Autodesk Fusion 360 part; units mm, degrees
sketch "Sketch1" plane through (0, 0, 0) normal (0, 0, 1) x (1, 0, 0)
  line L0 (50, 55) -> (66, 55) construction
  line L1 (50, 55) -> (34, 55) construction
  line L2 (50, 55) -> (50, 39) construction
  line L3 (50, 55) -> (50, 71) construction
  circle A0 centre (40.5, 55) radius 1.6
  circle A1 centre (50, 63) radius 1.6
  circle A2 centre (59.5, 55) radius 1.6
  circle A3 centre (50, 47) radius 1.6
  line L4 (65, 55) -> (66, 55)
  line L5 (35, 55) -> (34, 55)
  line L6 (50, 55) -> (46.1698, 51.7861) construction
  arc A4 (61.4907, 45.3582) -> (65, 55) centre (50, 55) ccw
  arc A5 (35, 55) -> (38.5093, 45.3582) centre (50, 55) ccw
  circle A6 centre (50, 55) radius 5
  line L7 (34, 55) -> (33.5, 55)
  line L8 (66, 55) -> (66.5, 55)
  circle A7 centre (50, 55) radius 15
  line L9 (50, 55) -> (53.8302, 51.7861) construction
  line L10 (61.4907, 45.3582) -> (62.2567, 44.7154) construction
  arc A8 (33.5, 55) -> (66.5, 55) centre (50, 55) ccw
  point P0 (59.5, 55)
  point P1 (50, 63)
  point P2 (50, 47)
  point P3 (40.5, 55)
  dimension "d23" = 30
  dimension "d25" = 8
  dimension "d26" = 8
  dimension "d27" = 9.5
  dimension "d28" = 9.5
  dimension "d29" = 3.2
  dimension "d30" = 3.2
  dimension "d31" = 3.2
  dimension "d32" = 3.2
  dimension "d33" = 140
  dimension "d34" = 80
  dimension "d41" = 10
  dimension "d44" = 33
extrude "Extrude7" add sketch "Sketch1" along normal blind 3 contours A4 A5 A7
extrude "Extrude8" add sketch "Sketch1" along normal blind 27 contours L4 L5 A4 A5 L7 L8 A7 A8
chamfer "Chamfer2" distance 0.5 distance2 2 1 edges at (45.3384, 56.8081, 3) measured on face at (42.065, 60.0544, 3)
chamfer "Chamfer3" distance 2 distance2 1 4 edges at (58.0083, 55.5786, 0) (48.5083, 47.5786, 0) (39.0083, 55.5786, 0) (48.5083, 63.5786, 0) measured on face at (60.434, 56.2991, 2) measured on face at (50.934, 48.2991, 2) measured on face at (41.434, 56.2991, 2) measured on face at (51.0587, 64.1997, 2)
fillet "Fillet1" radius 1.5 2 edges at (65, 55, 1.5) (35, 55, 1.5)
sketch "Sketch2" plane through (0, 0, 0) normal (0, 1, 0) x (1, 0, 0)
The model under review builds one solid part; all positions refer to its coordinate system, in mm. A direction names the side the tool comes from. Coordinates: 2 decimals unless noted, no trailing zeros. Write each loop counter-clockwise with the first axis right and the second up, starting at its lowest first coordinate (ties: lowest second). Pieces come first, ordered by that corner, then holes. Notation, with made-up numbers: (-18, 42.5) - (-14, 42.5) arc R23 cw to (-14, 51.5) - close; hole circle Ø10 at (86.25, -0.5). An arc over 180 degrees is marked (long way). Answer in a Markdown table with one row per item. Add a question column.
Q1. Consider section C-C on z = 19.75. Give the boundary of the cut face in (x, y).
Q2. To check wall thickness, follow line 1 along Y through (x, z) = (50, 2.6); line 2 along Y through (x, z) = (50, 0.35) (3 decimals); line 3 along Z through (x, y) = (58, 43.5). State the ranges of each line that lie inside material, in increasing order. Write a range as from..to.
Q3. Consider section A-A on x = 40.5. Give the boundary of the cut face in (y, z).
Q4. Clearance check with flat-ended pins moving along their axes: pin 1 (1.5 mm diameter, centred on y = 54.5, z = 18.5, fed in from +X); pin 2 (1.9 mm diameter, centred on x = 50, y = 47, fed in from +Z); pin 3 (6 mm diameter, centred on x = 55, z = 12.5, fed in from -Y); pin 4 (3.5 mm diameter, centred on x = 59.5, y = 55, fed in from +Z). State where each tip first meets the part, or that it passes through.
Q5. Draft analysis for pull direction Y (two halves, no side actions). For faces 1 (the face through (34.568, 55.382, 1.521)), 2 (the face through (53.4, 51, 0)), 3 (the face through (61.026, 54.519, 2.493)), 4 (the face through (49.349, 50.043, 0.493)), state which applies: +Y half, -Y half, draft (parallel to the pull), parting line (faces both ways), or undercut.
Q6. For faces 5 (the face through (57, 55, 3)), 6 (the face through (65.41, 55.4, 1.52)), list the 3-axis set-ups (+Z, -Z, +X, -X, +Y, -Y) from which the entire face can be reached by the end or side of a thin tool; tool diameter is ignored.
Q7. Consider section D-D on y = 47. Give the boundary of the cut face in (x, z).
Q8. Consider section B-B on y = 63. Give the boundary of the cut face in (x, z), then the cut area to 3 significant figures.
Answers below:
| question | item | result |
|---|---|---|
| 1 | outline | (33.5, 55) arc R16.5 ccw to (66.5, 55) - (65, 55) arc R15 cw to (61.49, 45.36) arc R15 cw to (38.51, 45.36) arc R15 cw to (35, 55) - close |
| 2 | line 1 | 38.5..45.4, 48.6..49.6, 60.4..61.4, 64.6..70 |
| 2 | line 2 | 38.5..44.575, 49.425..50, 60..60.575, 65.425..70 |
| 2 | line 3 | 0..3 |
| 3 | outline | (41.51, 0) - (52.4, 0) - (53.4, 2) - (53.4, 3) - (43.39, 3) - (43.39, 27) - (41.51, 27) - close; (56.6, 2) - (57.6, 0) - (66.61, 0) - (66.61, 3) - (56.6, 3) - close |
| 4 | pin 1 | x = 66.5 |
| 4 | pin 2 | through |
| 4 | pin 3 | y = 38.62 |
| 4 | pin 4 | z = 3 |
| 5 | face 1 | +Y half |
| 5 | face 2 | draft |
| 5 | face 3 | undercut |
| 5 | face 4 | undercut |
| 6 | face 5 | +Z, +Y |
| 6 | face 6 | +Z, -Z, +X, +Y |
| 7 | outline | (35.57, 0) - (47.4, 0) - (48.4, 2) - (48.4, 3) - (37.31, 3) - (37.31, 27) - (35.57, 27) - close; (51.6, 2) - (52.6, 0) - (64.43, 0) - (64.43, 27) - (62.69, 27) - (62.69, 3) - (51.6, 3) - close |
| 8 | outline | (37.31, 0) - (47.4, 0) - (48.4, 2) - (48.4, 3) - (37.31, 3) - close; (51.6, 2) - (52.6, 0) - (62.69, 0) - (62.69, 3) - (51.6, 3) - close |
| 8 | area | 64.5 mm² |
